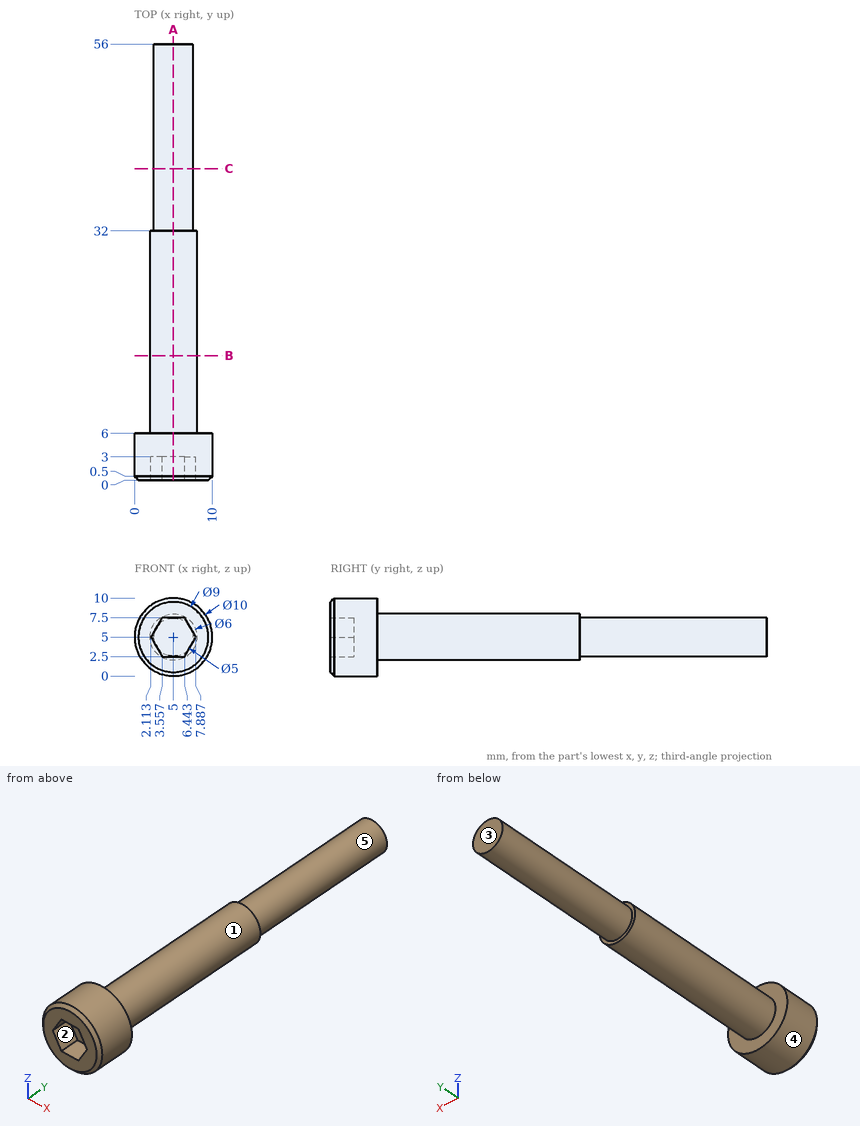
Drawing for the job (mm, zero at the part's lowest x, y, z). A direction names the side the tool comes from. Give positions to 0.01 mm unless a question says otherwise; leave off trailing zeros. Loops run counter-clockwise (first coordinate to the right, second up) from the corner with the lowest first, then second, coordinate; pieces in that order, holes last.
1) Band-saw the part on A-A on x = 5. List the corners of the cut face in (y, z).
Values follow:
outline: (0, 0.5) - (0.5, 0) - (6, 0) - (6, 2) - (32, 2) - (32, 2.5) - (56, 2.5) - (56, 7.5) - (32, 7.5) - (32, 8) - (6, 8) - (6, 10) - (0.5, 10) - (0, 9.5) - (0, 7.5) - (3, 7.5) - (3, 2.5) - (0, 2.5) - close
2) 3-axis set-ups, long thin cutter, end or side, ignore diameter. For the marked faces 4 and 5: which of +Z, -Z, +X, -X, +Y, -Y reach the whole face in a straight line?
Values follow:
face 4: +Y, -Y
face 5: +Y
3) Band-saw the part on C-C on y = 40. List the corners of the cut face in (x, z).
Values follow:
outline: circle Ø5 at (5, 5)
4) Probe line 1 along Y through (x, z) = (1.75, 3.75); line 2 along Y through (x, z) = (7, 3); line 3 along Z through (x, y) = (1, 3). List the from-to ranges inside material, lowest first.
Values follow:
line 1: y = 0 to 6
line 2: y = 0 to 32
line 3: z = 2 to 8
5) Two-plate mould, pull along X, no slides. Class the marked faces 1, 2 and 3: released by +X, released by -X, zero draft, split by the parting line, or undercut.
Values follow:
face 1: split by the parting line
face 2: undercut
face 3: zero draft
6) Drop flat-ended pins along their axis: P1, Ø4, axis at y = 10, z = 3, coming from the +X side; P2, Ø2, axis at y = 24.5, z = 8, coming from the -X side (1 decimal); P3, Ø2, axis at x = 5.5, z = 1.5, coming from the +Y side. Give the stop position or say it passes through.
Values follow:
P1: stops at x = 8
P2: stops at x = 2.8
P3: stops at y = 32
7) Band-saw the part on B-B on y = 16. List the corners of the cut face in (x, z).
Values follow:
outline: circle Ø6 at (5, 5)
